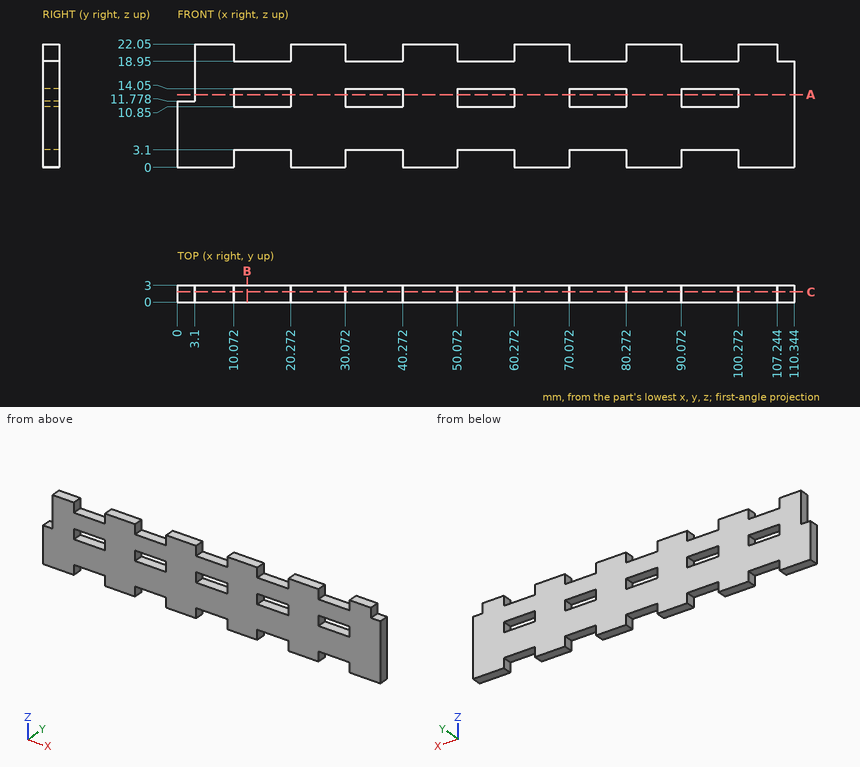
Print and shaded views of the part. All mm, measured from the part's lowest x, y and z. Coordinates: 2 decimals unless noted, no trailing zeros. Order: outer loops, then holes, each group sorted by start corner. A loop starts at its lowest first (then second) coordinate and runs counter-clockwise, first axis right, second up. Notation, with made-up numbers: (15.5, 24) -> (64.5, 24) arc R20 ccw to (64.5, 37) -> close; hole circle Ø3 at (14.5, 36.5). An arc over 180 degrees is marked (long way). Use one line per item in the form item = value. Start each with the question number.
1) Band-saw the part on C-C on y = 1.85. State how many separate pieces and enclosed holes the cut face has, then the cut area to 3 significant figures.
2) Band-saw the part on B-B on x = 12.5. Give the cut face in (y, z).
3) Band-saw the part on A-A on z = 13. Give the cut face in (x, y) (1 decimal), then the cut area to 3 significant figures.
4) Drop flat-ended pins along their axis: pin 1 (1.5 mm diameter, centred on y = 2, z = 20, fed in from -X); pin 2 (1 mm diameter, centred on y = 1.5, z = 6.5, fed in from -X); pin 3 (0.9 mm diameter, centred on x = 16, y = 2, fed in from +Z); pin 4 (0.9 mm diameter, centred on y = 1, z = 21, fed in from +X). Give the stop position or say it passes through.
5) Drill centre lines: L1, parallel to X at y = 2.6, z = 1 (1 decimal); L2, parallel to Z at x = 73, y = 0.5; L3, parallel to X at y = 0.5, z = 18.75 (1 decimal). Where is each one in solid material? Low to high. Write a range as [from, to].
Entries:
q1.separate_pieces = 1
q1.enclosed_holes = 5
q1.area = 1,910 mm2
q2.outline = (0, 3.1) -> (3, 3.1) -> (3, 10.85) -> (0, 10.85) -> close; (0, 14.05) -> (3, 14.05) -> (3, 18.95) -> (0, 18.95) -> close
q3.outline = (3.1, 0) -> (10.1, 0) -> (10.1, 3) -> (3.1, 3) -> close; (20.3, 0) -> (30.1, 0) -> (30.1, 3) -> (20.3, 3) -> close; (40.3, 0) -> (50.1, 0) -> (50.1, 3) -> (40.3, 3) -> close; (60.3, 0) -> (70.1, 0) -> (70.1, 3) -> (60.3, 3) -> close; (80.3, 0) -> (90.1, 0) -> (90.1, 3) -> (80.3, 3) -> close; (100.3, 0) -> (110.3, 0) -> (110.3, 3) -> (100.3, 3) -> close
q3.area = 169 mm2
q4.pin_1 = 3.1
q4.pin_2 = 0
q4.pin_3 = 18.95
q4.pin_4 = 107.24
q5.L1 = [0, 10.1], [20.3, 30.1], [40.3, 50.1], [60.3, 70.1], [80.3, 90.1], [100.3, 110.3]
q5.L2 = [3.1, 10.85], [14.05, 18.95]
q5.L3 = [3.1, 110.3]
